from build123d import *

# Parameters (mm, degrees)
FILLET1_R                = 2.5
BOSS_EXTRUDE1_DEPTH      = 1.5
FILLET2_R                = 4
CIRPATTERN1_COUNT        = 5
FILLET2_OF_CIRPATTERN1_R = 4
CUT_EXTRUDE1_START       = -29.0000001
SKETCH4_R                = 10
CUT_EXTRUDE1_DEPTH       = 30.0000001
BOSS_EXTRUDE2_DEPTH      = 12
SKETCH6_W                = 1.75
SKETCH6_H                = 24
BOSS_EXTRUDE3_DEPTH      = 8.5
CIRPATTERN2_COUNT        = 5


with BuildPart() as part:
    # Sketch2 → Revolve1 (revolve)
    with BuildSketch(Plane(origin=(0, 0, 0), x_dir=(0, 0, -1), z_dir=(1, 0, 0))):
        Polygon((2.5, 44.5), (2.5, 37.5), (-10.5, 37.5), (-10.5, 26), (-18, 26), (-18, 22.5), (-10.5, 22.5), (-10.5, 9.5), (0, 9.5), (0, 11.5), (-8.5, 11.5), (-8.5, 35.5), (4.5, 35.5), (4.5, 44.5), align=None)
    revolve(axis=Axis((0, 0, -45.438153482), (0, 0, 1)))

    # Fillet1
    fillet1_edges = [part.edges().sort_by_distance(p)[0] for p in [
        (0, -37.5, 10.5),
    ]]
    fillet(fillet1_edges, radius=FILLET1_R)

    # Sketch3 → Boss-Extrude1 (add, symmetric)
    with BuildSketch(Plane(origin=(0, 0, 0), x_dir=(0, 0, -1), z_dir=(1, 0, 0))):
        with BuildLine():
            Line((2.5, 40.7), (-19, 40.7))
            ThreePointArc((-19, 40.7), (-22.181980515, 39.381980515), (-23.5, 36.2))
            Line((-23.5, 36.2), (-23.5, 28.592964966))
            Line((-23.5, 28.592964966), (-10.5, 10.7))
            Line((-10.5, 10.7), (-10.5, 33.460767767))
            Line((-10.5, 33.460767767), (-6.918763004, 36.95))
            Line((-6.918763004, 36.95), (2.5, 36.95))
            Line((2.5, 36.95), (2.5, 40.7))
        make_face()
    boss_extrude1 = extrude(amount=BOSS_EXTRUDE1_DEPTH, both=True)

    # Fillet2
    fillet2_edges = [part.edges().sort_by_distance(p)[0] for p in [
        (0, 28.592964966, 23.5),
    ]]
    fillet(fillet2_edges, radius=FILLET2_R)

    # CirPattern1: Boss-Extrude1 ×5 about axis
    cirpattern1_axis = Axis((0, 0, 0), (0, 0, 1))
    for i in range(1, CIRPATTERN1_COUNT):
        add(boss_extrude1.rotate(cirpattern1_axis, i * 360 / CIRPATTERN1_COUNT))

    # Fillet2 of CirPattern1
    fillet2_of_cirpattern1_edges = [part.edges().sort_by_distance(p)[0] for p in [
        (-27.193525651, 8.835712094, 23.5),
        (-16.806523126, -23.132194577, 23.5),
        (16.806523126, -23.132194577, 23.5),
        (27.193525651, 8.835712094, 23.5),
    ]]
    fillet(fillet2_of_cirpattern1_edges, radius=FILLET2_OF_CIRPATTERN1_R)

    # Sketch4 → Cut-Extrude1 (cut)
    with BuildSketch(Plane(origin=(0, 0, -4.5), x_dir=(-1, 0, 0), z_dir=(0, 0, -1)).offset(CUT_EXTRUDE1_START)):
        with Locations((0, -52)):
            Circle(SKETCH4_R)
    cut_extrude1 = extrude(amount=CUT_EXTRUDE1_DEPTH, mode=Mode.SUBTRACT)

    # Sketch5 → Boss-Extrude2 (add)
    with BuildSketch(Plane(origin=(0, 0, 8.5), x_dir=(-1, 0, 0), z_dir=(0, 0, -1))):
        with BuildLine():
            Line((-2.997320764, -35.373239437), (0, -37.103743386))
            Line((0, -37.103743386), (2.997320764, -35.373239437))
            ThreePointArc((2.997320764, -35.373239437), (0, -32.5), (-2.997320764, -35.373239437))
        make_face()
    boss_extrude2 = extrude(amount=BOSS_EXTRUDE2_DEPTH)

    # Sketch6 → Boss-Extrude3 (add)
    with BuildSketch(Plane(origin=(0, 0, 8.5), x_dir=(-1, 0, 0), z_dir=(0, 0, -1))):
        with Locations((0, -22.75)):
            Rectangle(SKETCH6_W, SKETCH6_H)
    boss_extrude3 = extrude(amount=BOSS_EXTRUDE3_DEPTH)

    # CirPattern2: Cut-Extrude1, Boss-Extrude2, Boss-Extrude3 ×5 about axis
    cirpattern2_axis = Axis((0, 0, 0), (0, 0, 1))
    for i in range(1, CIRPATTERN2_COUNT):
        add(cut_extrude1.rotate(cirpattern2_axis, i * 360 / CIRPATTERN2_COUNT), mode=Mode.SUBTRACT)
        add(boss_extrude2.rotate(cirpattern2_axis, i * 360 / CIRPATTERN2_COUNT))
        add(boss_extrude3.rotate(cirpattern2_axis, i * 360 / CIRPATTERN2_COUNT))


solid = part.part
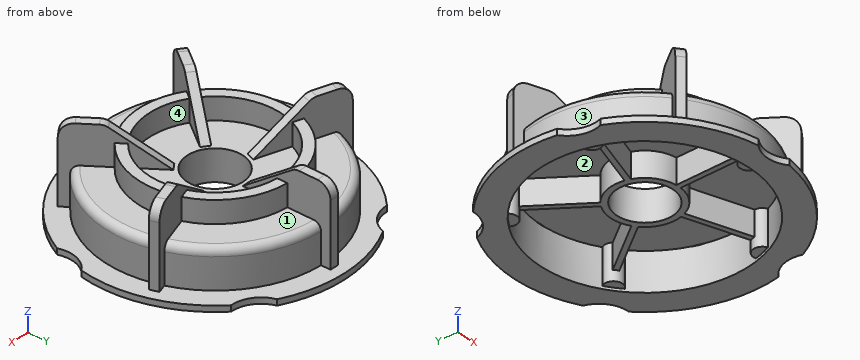
Input: part model. Units: mm. Frame: model coordinates. Face numbers are marked on the shaded views. A direction names the side the tool comes from. Coordinates: 2 decimals unless noted, no trailing zeros.
Q1. Cut plane B-B (z = 2). Give the number of separate pieces and of enclosed holes in the cut face, then the cut area to 3 significant figures.
Q2. Contact query for flat-ended pins moving along their axis: pin 1 (2.5 mm diameter, centred on y = -23, z = 5, fed in from -X); pin 2 (1.5 mm diameter, centred on y = -3.5, z = 20.5, fed in from -X); pin 3 (6 mm diameter, centred on x = -3, z = 8, fed in from -Y); pin 4 (8 mm diameter, centred on x = 21.5, y = -11.5, fed in from -Z). Output: stop coordinate, or through.
Q3. Material intervals for line 1 (X direction, y = 0, z = 7.25); line 2 (X direction, y = 2, z = 6.75); line 3 (Y direction, x = -4.5, z = 7.75), sorted ascending.
Q4. Set-up query: the marked faces 1, 2, 3 and 4. Return all of +Z, -Z, +X, -X, +Y, -Y with unobstructed straight access to the full face (end or side cutting, diameter ignored); none if empty.
Working result:
1. separate pieces: 1
1. enclosed holes: 6
1. area: 892 mm2
2. pin 1: stops at x = -30.55
2. pin 2: passes through
2. pin 3: stops at y = -37.5
2. pin 4: stops at z = 0
3. line 1: x = -37.5 to -35.5, -11.5 to -9.5, 9.5 to 11.5, 35.5 to 37.5
3. line 2: x = -37.45 to -35.44, -11.32 to -9.29, 9.29 to 11.32, 35.44 to 37.45
3. line 3: y = -37.23 to -35.21, -10.58 to -8.37, 8.37 to 10.58, 35.21 to 37.23
4. face 1: +Z, +Y
4. face 2: -Z
4. face 3: +Z, -X
4. face 4: +Z
